from build123d import *
from build123d.topology import SkipClean

# Parameters (mm, degrees)
CROQUIS1_R                 = 2
CROQUIS1_R_2               = 2.000000000000003
SALIENTE_EXTRUIR1_DEPTH    = 20
CORTAR_EXTRUIR1_DEPTH      = 44.68065933568311
CORTAR_EXTRUIR2_DEPTH      = 44.68065933568311
CORTAR_EXTRUIR2_DEPTH_BACK = 44.68065933568311
BOSS_EXTRUDE2_START        = -16
BOSS_EXTRUDE2_DEPTH        = 5
CHAFL_N1_SIZE              = 2
CHAFL_N2_SIZE              = 3
CORTAR_EXTRUIR3_DEPTH      = 46.12195091942049
CORTAR_EXTRUIR3_DEPTH_BACK = 46.12195091942049
CROQUIS4_W                 = 13
CROQUIS4_H                 = 8.000000000000007
BOSS_EXTRUDE1_START        = -12.5
SKETCH4_R                  = 2.000000000000003
BOSS_EXTRUDE1_DEPTH        = 20
CUT_EXTRUDE2_START         = -12.5
SKETCH6_R                  = 6.150000000000001
CUT_EXTRUDE2_DEPTH         = 8
CUT_EXTRUDE1_START         = -20.5
CUT_EXTRUDE1_DEPTH         = 32.38680424515073
CUT_EXTRUDE3_START         = 20
SKETCH7_R                  = 2.500000000000002
CUT_EXTRUDE3_DEPTH         = 1
CHAMFER2_SIZE              = 3
CUT_EXTRUDE4_DEPTH         = 52.88680424515073
CUT_EXTRUDE4_DEPTH_BACK    = 52.88680424515073
SKETCH9_R                  = 1.1750000000000003
FILLET1_R                  = 2


with BuildPart() as part:
    # Croquis1 → Saliente-Extruir1 (new, symmetric)
    with BuildSketch(Plane.XY):
        with BuildLine():
            Line((0, 8), (30, 8))
            ThreePointArc((30, 8), (38, 0), (30, -8))
            Line((30, -8), (0, -8))
            ThreePointArc((0, -8), (-8, 9.8e-16), (0, 8))
        make_face()
        Circle(CROQUIS1_R, mode=Mode.SUBTRACT)
        with Locations((30, 0)):
            Circle(CROQUIS1_R_2, mode=Mode.SUBTRACT)
    extrude(amount=SALIENTE_EXTRUIR1_DEPTH, both=True)

    # Croquis2 → Cortar-Extruir1 (cut, symmetric)
    with BuildSketch(Plane(origin=(0, 0, 0), x_dir=(1, 0, 0), z_dir=(0, 1, 0))):
        Polygon((-8, 16), (8.77460379211011, 16), (18.02448398763881, 20), (-8, 20), align=None)
    cortar_extruir1 = extrude(amount=CORTAR_EXTRUIR1_DEPTH, both=True, mode=Mode.SUBTRACT)

    # Simetría1: Cortar-Extruir1 across plane
    add(cortar_extruir1.mirror(Plane.XY), mode=Mode.SUBTRACT)

    # Croquis3 → Cortar-Extruir2 (cut, two sides: drawn at the far end of the back side and taken through both)
    with BuildSketch(Plane(origin=(0, 0, 0), x_dir=(1, 0, 0), z_dir=(0, 1, 0)).offset(-CORTAR_EXTRUIR2_DEPTH_BACK)):
        Polygon((49.99999999999999, -12.499999999999998), (9.999999999999998, -12.500000000000004), (9.999999999999998, 12.499999999999996), (49.99999999999999, 12.500000000000002), align=None)
    extrude(amount=CORTAR_EXTRUIR2_DEPTH + CORTAR_EXTRUIR2_DEPTH_BACK, mode=Mode.SUBTRACT)

    # Sketch8 → Boss-Extrude2 (add)
    with SkipClean():  # the faces are left unmerged after this step: merging them gives an invalid solid
        with BuildSketch(Plane.XY.offset(BOSS_EXTRUDE2_START)):
            with BuildLine():
                ThreePointArc((-3.7e-16, -2), (-0.5344767521565125, -1.9272609064172463), (-1.0300761498201043, -1.714334601404227))
                Line((-1.0300761498201039, -1.7143346014042276), (-7.918066759935976, -13.177876048443173))
                Line((-7.918066759935977, -13.177876048443173), (-6.789375757901606, -13.856062022616376))
                Line((-6.789375757901606, -13.856062022616376), (0, -8))
                Line((0, -8), (0, -2))
            make_face()
        extrude(amount=BOSS_EXTRUDE2_DEPTH)

    # Chaflán1
    chafl_n1_edges = [part.edges().sort_by_distance(p)[0] for p in [
        (38, -4e-16, 20),
        (24.012241993819405, 8, 20),
        (24.012241993819405, -8, -20),
        (24.012241993819405, 8, -20),
        (24.012241993819405, -8, 20),
        (38, -4e-16, -20),
    ]]
    chamfer(chafl_n1_edges, length=CHAFL_N1_SIZE)

    # Chaflán2
    chafl_n2_edges = [part.edges().sort_by_distance(p)[0] for p in [
        (9.999999999999998, 0, -12.499999999999996),
        (9.999999999999998, 0, 12.500000000000004),
    ]]
    chamfer(chafl_n2_edges, length=CHAFL_N2_SIZE)

    # Croquis4 → Cortar-Extruir3 (cut, two sides: drawn at the far end of the back side and taken through both)
    with SkipClean():  # the faces are left unmerged after this step: merging them gives an invalid solid
        with BuildSketch(Plane(origin=(0, 0, 0), x_dir=(1, 0, 0), z_dir=(0, 1, 0)).offset(-CORTAR_EXTRUIR3_DEPTH_BACK)):
            with Locations((-1.5, 0)):
                Rectangle(CROQUIS4_W, CROQUIS4_H)
        extrude(amount=CORTAR_EXTRUIR3_DEPTH + CORTAR_EXTRUIR3_DEPTH_BACK, mode=Mode.SUBTRACT)

    # Sketch4 → Boss-Extrude1 (add)
    with SkipClean():  # the faces are left unmerged after this step: merging them gives an invalid solid
        with BuildSketch(Plane.XY.offset(BOSS_EXTRUDE1_START)):
            with BuildLine():
                Line((22, 6.000000000000003), (22.000000000000004, -6.000000000000014))
                Line((22.000000000000004, -6.000000000000014), (35.291502622129165, -6.000000000000012))
                ThreePointArc((35.291502622129165, -6.000000000000012), (38, 4.44e-15), (35.29150262212916, 6.000000000000019))
                Line((35.29150262212916, 6.000000000000019), (22, 6.000000000000003))
            make_face()
            with Locations(Location((30, 0, 0), (0, 0, 180))):
                Circle(SKETCH4_R, mode=Mode.SUBTRACT)
        extrude(amount=-BOSS_EXTRUDE1_DEPTH)

    # Sketch6 → Cut-Extrude2 (cut)
    with SkipClean():  # the faces are left unmerged after this step: merging them gives an invalid solid
        with BuildSketch(Plane.XY.offset(CUT_EXTRUDE2_START)):
            with Locations(Location((30, 0, 0), (0, 0, 282.680383492))):
                Circle(SKETCH6_R)
        extrude(amount=-CUT_EXTRUDE2_DEPTH, mode=Mode.SUBTRACT)

    # Sketch5 → Cut-Extrude1 (cut, through all)
    with SkipClean():  # the faces are left unmerged after this step: merging them gives an invalid solid
        with BuildSketch(Plane.XY.offset(CUT_EXTRUDE1_START)):
            with BuildLine():
                Line((26.26904837876446, 5.2), (33.73095162123554, 5.2))
                ThreePointArc((33.73095162123554, 5.2), (36.400000000000006, 7.1e-16), (33.73095162123554, -5.199999999999998))
                Line((33.73095162123554, -5.199999999999998), (26.26904837876446, -5.2))
                ThreePointArc((26.26904837876446, -5.2), (23.59999999999999, 7.8e-16), (26.26904837876446, 5.2))
            make_face()
        extrude(amount=-CUT_EXTRUDE1_DEPTH, mode=Mode.SUBTRACT)

    # Sketch7 → Cut-Extrude3 (cut)
    with SkipClean():  # the faces are left unmerged after this step: merging them gives an invalid solid
        with BuildSketch(Plane.XY.offset(CUT_EXTRUDE3_START)):
            with Locations((30, 0)):
                Circle(SKETCH7_R)
        extrude(amount=-CUT_EXTRUDE3_DEPTH, mode=Mode.SUBTRACT)

    # Chamfer2
    chamfer2_edges = [part.edges().sort_by_distance(p)[0] for p in [
        (22.000000000000004, -6.000000000000014, -26.25),
        (22, 6.000000000000003, -26.25),
    ]]
    chamfer(chamfer2_edges, length=CHAMFER2_SIZE)

    # Sketch9 → Cut-Extrude4 (cut, two sides: drawn at the far end of the back side and taken through both)
    with BuildSketch(Plane(origin=(0, 0, 0), x_dir=(1, 0, 0), z_dir=(0, 1, 0)).offset(-CUT_EXTRUDE4_DEPTH_BACK)):
        with Locations(Location((2, 10.923187610000003, 0), (0, 0, 270))):
            Circle(SKETCH9_R)
        with Locations(Location((2, -9.076812389999997, 0), (0, 0, 270))):
            Circle(SKETCH9_R)
    extrude(amount=CUT_EXTRUDE4_DEPTH + CUT_EXTRUDE4_DEPTH_BACK, mode=Mode.SUBTRACT)

    # Fillet1
    fillet1_edges = [part.edges().sort_by_distance(p)[0] for p in [
        (5, 0, -4.0000000000000036),
        (5, 0, 4.0000000000000036),
    ]]
    fillet(fillet1_edges, radius=FILLET1_R)


solid = part.part
Verification items for the finished model (mm, model axes). A direction names the side the tool comes from. Coordinates: 2 decimals unless noted, no trailing zeros. Order: outer loops, then holes, each group sorted by start corner. A loop starts at its lowest first (then second) coordinate and runs counter-clockwise, first axis right, second up.
Item 1: Release check for a two-part mould opening along Z. For faces 1 (the face through (11.5, -0.1, 11)), 2 (the face through (24, -7, -19)), 3 (the face through (31.908, 0.601, 15.704)), 4 (the face through (3.165, -0.112, 8.924)) record: +Z half, -Z half, draft (parallel to the pull), parting line (faces both ways), or undercut.
Filled in:
face 1: undercut
face 2: -Z half
face 3: draft
face 4: undercut
Item 2: Section check B-B, the plane y = 0. Give the number of separate pieces and of enclosed holes in the cut face, then the cut area to 3 significant figures.
Filled in:
separate pieces: 5
enclosed holes: 0
area: 690 mm2
Item 3: Depth check by flat-ended pin: pin 1 (0.9 mm diameter, centred on x = 35, y = -2, fed in from -Z); pin 2 (8 mm diameter, centred on x = 5, y = 5, fed in from -Z); pin 3 (3 mm diameter, centred on x = 16, z = -20, fed in from -Y); pin 4 (1.5 mm diameter, centred on x = 31, y = 0.5, fed in from +Z) (1 decimal). Enter the tip coordinate at first touch or a pass-through.
Filled in:
pin 1: stops at z = 12.5
pin 2: stops at z = -16.1
pin 3: stops at y = -7.5
pin 4: passes through
Item 4: Section check C-C, the plane x = 7.5. Enter the section's corners in (y, z), then the cut area to 3 significant figures.
Filled in:
outline: (-8, -16) - (8, -16) - (8, 16) - (-8, 16) - close
area: 512 mm2
Item 5: Section check A-A, the plane x = -5. Enter the section's corners in (y, z) (3 decimals), then the cut area to 3 significant figures.
Filled in:
outline: (-12.313, -16) - (-8.321, -16) - (-8.321, -11) - (-12.313, -11) - close; (-6.245, -16) - (6.245, -16) - (6.245, -4) - (-6.245, -4) - close; (-6.245, 4) - (6.245, 4) - (6.245, 16) - (-6.245, 16) - close
area: 320 mm2
Item 6: Material ranges on L1, parallel to X at y = 0, z = 13.75; L2, parallel to X at y = 0, z = -15; L3, parallel to Y at x = 30, z = 17.5, recorded low to high.
Filled in:
L1: x = -8 to -2, 2 to 28, 32 to 38
L2: x = -8 to -2, 2 to 23.85, 36.15 to 38
L3: y = -8 to -2, 2 to 8
Item 7: Access from +Z, -Z, +X, -X, +Y, -Y to the whole of each face (thin tool, end or side, straight path). Record for faces 5 (the face through (-8, 0, 10)), 6 (the face through (9, -8, 0)), 7 (the face through (23, 0, -12.5)), 8 (the face through (23, 7, -19)), 9 (the face through (5, 0, 0)).
Filled in:
face 5: +Z, -X
face 6: +Z, -Z, +X, -Y
face 7: +X, +Y, -Y
face 8: -Z, +X, -X, +Y
face 9: -X, +Y, -Y
